Autodesk Inventor part; units mm, degrees
ref_plane "YZ Plane" through (0, 0, 0) normal (1, 0, 0) x (0, 1, 0)
ref_plane "XZ Plane" through (0, 0, 0) normal (0, 1, 0) x (-1, 0, 0)
ref_plane "XY Plane" through (0, 0, 0) normal (0, 0, 1) x (1, 0, 0)
sketch "Sketch1" plane through (0, 0, 0) normal (0, 0, 1) x (1, 0, 0)
  line L0 (0, 0) -> (-25.4, 0)
  line L1 (-25.4, 0) -> (-25.4, 76.2)
  line L2 (-25.4, 76.2) -> (0, 76.2)
  line L3 (0, 76.2) -> (0, 0)
  line L4 (-25.4, 7.874) -> (-49.5487, 0)
  line L5 (-49.5487, 0) -> (-73.1707, 72.4461)
  line L6 (-73.1707, 72.4461) -> (-49.022, 80.3201)
  line L7 (-49.022, 80.3201) -> (-25.4, 7.874)
  circle A0 centre (-24.1487, 0) radius 24.1487
  line L8 (-49.5487, 0) -> (-47.1078, -7.4861)
  dimension "d0" = 25.4
  dimension "d1" = 76.2
  dimension "d3" = 25.4
  dimension "d4" = 7.874
  dimension "d5" = 76.2
extrude "Extrusion1" add sketch "Sketch1" along normal blind 3.175 contours A0 L4 L1 L0 | A0 L1 L2 L3 | L0 L1 A0 | L8 L4 A0 | L4 A0 L7 | L4 L5 L6 L7 A0
fillet "Fillet1" radius 6.35 1 edges at (-25.4, 7.874, 1.5875)
sketch "Sketch2" plane through (0, 0, 3.175) normal (0, 0, 1) x (1, 0, 0)
  line L0 (0, 76.2) -> (-25.4, 76.2)
  line L1 (-25.4, 76.2) -> (-25.4, 47.8326)
  arc A0 (-37.7872, 45.8641) -> (-25.4, 47.8326) centre (-31.75, 47.8326) ccw
  line L2 (-37.7872, 45.8641) -> (-49.022, 80.3201)
  line L3 (-49.022, 80.3201) -> (-73.1707, 72.4461)
  line L4 (-73.1707, 72.4461) -> (-47.1078, -7.4861)
  arc A1 (-47.1078, -7.4861) -> (0, 0) centre (-24.1487, 0) ccw
  line L5 (0, 0) -> (0, 76.2)
  circle A2 centre (-12.7, 63.5) radius 2.5527
  circle A3 centre (-12.7, 38.1) radius 2.5527
  circle A4 centre (-12.7, 12.7) radius 2.5527
  circle A5 centre (-57.1594, 64.3088) radius 2.5527
  circle A6 centre (-49.2854, 40.1601) radius 2.5527
  circle A7 centre (-41.4114, 16.0114) radius 2.5527
  dimension "d9" = 5.1054
  dimension "d10" = 12.7
  dimension "d11" = 12.7
  dimension "d14" = 25.4
  dimension "d19" = 5.1054
  dimension "d20" = 12.7
  dimension "d21" = 12.7
  dimension "d24" = 25.4
extrude "Extrusion2" cut sketch "Sketch2" against normal blind 3.175 contours A2 | A3 | A4 | A5 | A6 | A7
properties part number "Top_angled_gusset"
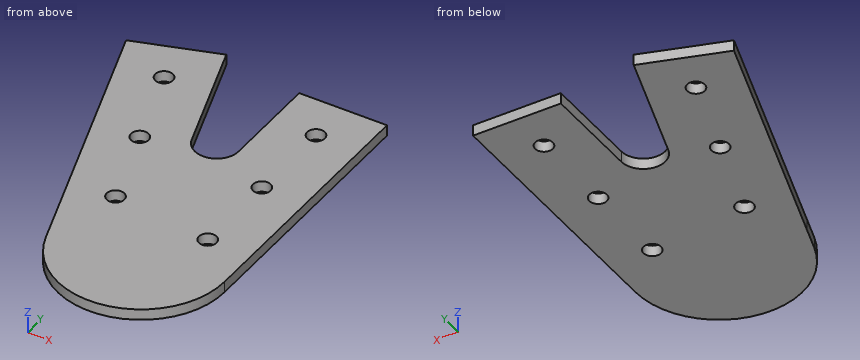
Can you work these out from the model? Positions are in its coordinate system, mm. Give positions to 0.01 mm unless a question says otherwise; leave off trailing zeros. Order: outer loops, then holes, each group sorted by start corner. A loop starts at its lowest first (then second) coordinate and runs counter-clockwise, first axis right, second up. Notation, with made-up numbers: M 23.25,58 L 57.25,58 A30 cw 57.25,96 Z; hole C 82.5,80.25 d4. An arc over 180 degrees is marked long. Write item = value, one per line. Start each with the question number.
Q1. Suppose I cut it at C-C (x = -29). Write out the boundary of the cut face in (y, z) (3 decimals).
Q2. Suppose I cut it at B-B (z = 1.4). Write out the boundary of the cut face in (x, y).
Q3. Will these pins go through, and if not, where does the flat tip stop? pin 1 Ø8 at (x, y) = (-49.29, 40.16) entering from -Z; pin 2 Ø1 at (y, z) = (68.5, 1) entering from -X; pin 3 Ø1.5 at (x, z) = (-22, 1) entering from +Y; pin 4 Ø4.5 at (x, y) = (-12.7, 63.5) entering from -Z.
Q4. Suppose I cut it at D-D (y = -11). Write out the boundary of the cut face in (x, z) (3 decimals).
Q5. I need wall thicknesses on probe 1 along Y at (x, z) = (-12.7, 1.05); probe 2 along Y at (x, z) = (-12, 1.4); probe 3 along X at (y, z) = (36, 2.9). Which ranges of each line are inside material? Lowest first, please. Write a range as [from, to].
Q6. Suppose I cut it at A-A (x = -12.7). Write out the boundary of the cut face in (y, z) (3 decimals), plus the area to 3 significant figures.
Check result:
q1.outline = M -23.656,0 L 42.109,0 L 42.109,3.175 L -23.656,3.175 Z
q2.outline = M -73.17,72.45 L -49.55,0 L -47.11,-7.49 A24.15 ccw 0,0 L 0,76.2 L -25.4,76.2 L -25.4,47.83 A6.35 cw -37.79,45.86 L -49.02,80.32 Z; hole C -57.16,64.31 d5.11; hole C -49.29,40.16 d5.11; hole C -41.41,16.01 d5.11; hole C -12.7,12.7 d5.11; hole C -12.7,38.1 d5.11; hole C -12.7,63.5 d5.11
q3.pin_1 = 0
q3.pin_2 = -72.05
q3.pin_3 = 76.2
q3.pin_4 = through
q4.outline = M -45.647,0 L -2.651,0 L -2.651,3.175 L -45.647,3.175 Z
q5.probe_1 = [-21.26, 10.15], [15.25, 35.55], [40.65, 60.95], [66.05, 76.2]
q5.probe_2 = [-20.87, 10.25], [15.15, 35.65], [40.55, 61.05], [65.95, 76.2]
q5.probe_3 = [-61.29, -14.15], [-11.25, 0]
q6.outline = M -21.262,0 L 10.147,0 L 10.147,3.175 L -21.262,3.175 Z; M 15.253,0 L 35.547,0 L 35.547,3.175 L 15.253,3.175 Z; M 40.653,0 L 60.947,0 L 60.947,3.175 L 40.653,3.175 Z; M 66.053,0 L 76.2,0 L 76.2,3.175 L 66.053,3.175 Z
q6.area = 261 mm2
